from build123d import *

# Parameters (mm, degrees)
SKETCH2_W                       = 42.4
SKETCH2_H                       = 76
SKETCH2_W_2                     = 38.4
SKETCH2_H_2                     = 72
BOSS_EXTRUDE4_DEPTH             = 32
SKETCH1_W                       = 42.4
SKETCH1_H                       = 30
SKETCH1_R                       = 3
BOSS_EXTRUDE1_DEPTH             = 2
SKETCH4_W                       = 56
SKETCH4_H                       = 30
SKETCH4_R                       = 1
BOSS_EXTRUDE5_DEPTH             = 2
SKETCH5_R                       = 1
CUT_EXTRUDE1_DEPTH              = 2
SKETCH9_W                       = 20
SKETCH9_H                       = 1
SKETCH11_W                      = 4.25
SKETCH11_H                      = 3
BOSS_EXTRUDE7_DEPTH             = 25
BOSS_EXTRUDE7_DIRECTION_2_REACH = 97.707
SKETCH12_R                      = 2
CUT_EXTRUDE2_DEPTH              = 25
CHAMFER1_SIZE                   = 1
BOSS_EXTRUDE8_DEPTH             = 2


with BuildPart() as part:
    # Sketch2 → Boss-Extrude4 (new body)
    with BuildSketch(Plane(origin=(0, 0, 0), x_dir=(1, 0, 0), z_dir=(0, 1, 0))):
        with Locations((19.2, 36)):
            Rectangle(SKETCH2_W, SKETCH2_H)
        with Locations((19.2, 36)):
            Rectangle(SKETCH2_W_2, SKETCH2_H_2, mode=Mode.SUBTRACT)
    extrude(amount=BOSS_EXTRUDE4_DEPTH)



with BuildPart() as body_2:
    # Sketch1 → Boss-Extrude1 (new body)
    with BuildSketch(Plane(origin=(0, 32, 0), x_dir=(1, 0, 0), z_dir=(0, 1, 0))):
        with Locations((19.2, 13)):
            Rectangle(SKETCH1_W, SKETCH1_H)
        with Locations(Location((4.2, 3, 0), (0, 0, 270))):
            Circle(SKETCH1_R, mode=Mode.SUBTRACT)
        with Locations(Location((34.2, 3, 0), (0, 0, 90))):
            Circle(SKETCH1_R, mode=Mode.SUBTRACT)
        with Locations(Location((34.2, 23, 0), (0, 0, 270))):
            Circle(SKETCH1_R, mode=Mode.SUBTRACT)
        with Locations(Location((4.2, 23, 0), (0, 0, 90))):
            Circle(SKETCH1_R, mode=Mode.SUBTRACT)
    extrude(amount=BOSS_EXTRUDE1_DEPTH)


with BuildPart() as part_1:
    add(part.part)

    add(body_2.part)  # Boss-Extrude5 merges body 2
    # Sketch4 → Boss-Extrude5 (add)
    with BuildSketch(Plane(origin=(0, 32, 0), x_dir=(1, 0, 0), z_dir=(0, 1, 0))):
        with Locations((19.2, 43)):
            Rectangle(SKETCH4_W, SKETCH4_H)
        with Locations(Location((-3.8, 33, 0), (0, 0, 270))):
            Circle(SKETCH4_R, mode=Mode.SUBTRACT)
        with Locations(Location((-3.8, 53, 0), (0, 0, 90))):
            Circle(SKETCH4_R, mode=Mode.SUBTRACT)
        with Locations(Location((42.2, 53, 0), (0, 0, 270))):
            Circle(SKETCH4_R, mode=Mode.SUBTRACT)
        with Locations(Location((42.2, 33, 0), (0, 0, 90))):
            Circle(SKETCH4_R, mode=Mode.SUBTRACT)
    extrude(amount=BOSS_EXTRUDE5_DEPTH)

    # Sketch5 → Cut-Extrude1 (cut)
    with BuildSketch(Plane.ZY.offset(2)):
        with Locations((-7.7, 5)):
            Circle(SKETCH5_R)
        with Locations((-7.7, 27)):
            Circle(SKETCH5_R)
        with Locations((-64.3, 27)):
            Circle(SKETCH5_R)
        with Locations((-64.3, 5)):
            Circle(SKETCH5_R)
    extrude(amount=-CUT_EXTRUDE1_DEPTH, mode=Mode.SUBTRACT)

    # Sketch9 → Revolve1 (revolve)
    with BuildSketch(Plane(origin=(0, 0, 0), x_dir=(0, 0, -1), z_dir=(1, 0, 0))):
        with Locations((46, 0.5)):
            Rectangle(SKETCH9_W, SKETCH9_H)
        with Locations((26, 0.5)):
            Rectangle(SKETCH9_W, SKETCH9_H)
    revolve1 = revolve(axis=Axis((0, 1, -56), (0, 0, 1)))

    # Mirror1: Revolve1 across plane
    add(revolve1.mirror(Plane(origin=(19.2, 0, 0), x_dir=(0, 0, 1), z_dir=(1, 0, 0))))

    # Sketch11 → Boss-Extrude7 (add)
    with BuildSketch(Plane(origin=(0, 0, -74), x_dir=(-1, 0, 0), z_dir=(0, 0, -1))):
        Polygon((-14.95, 0), (2, 0), (2, 2), (-40.4, 2), (-40.4, 0), (-23.45, 0), (-19.2, 0), align=None)
        with Locations((-21.325, -1.5)):
            Rectangle(SKETCH11_W, SKETCH11_H)
        with Locations((-17.075, -1.5)):
            Rectangle(SKETCH11_W, SKETCH11_H)
    extrude(amount=BOSS_EXTRUDE7_DEPTH)

    # Boss-Extrude7 direction 2: up to this face of the body (flat: up to its plane)
    boss_extrude7_direction_2_end = Plane(part_1.part.faces().sort_by_distance((19.2, 16, -72))[0])
    # Sketch11 → Boss-Extrude7 direction 2 (add, up to the picked face)
    with BuildSketch(Plane(origin=(0, 0, -74), x_dir=(-1, 0, 0), z_dir=(0, 0, -1)), mode=Mode.PRIVATE) as boss_extrude7_direction_2_sk1:
        Polygon((-14.95, 0), (2, 0), (2, 2), (-40.4, 2), (-40.4, 0), (-23.45, 0), (-19.2, 0), align=None)
    boss_extrude7_direction_2_tool1 = split(extrude(boss_extrude7_direction_2_sk1.sketch, amount=-BOSS_EXTRUDE7_DIRECTION_2_REACH, mode=Mode.PRIVATE), bisect_by=boss_extrude7_direction_2_end, keep=Keep.BOTH, mode=Mode.PRIVATE)
    # Sketch11 → Boss-Extrude7 direction 2 (add, up to the picked face)
    with BuildSketch(Plane(origin=(0, 0, -74), x_dir=(-1, 0, 0), z_dir=(0, 0, -1)), mode=Mode.PRIVATE) as boss_extrude7_direction_2_sk2:
        with Locations((-21.325, -1.5)):
            Rectangle(SKETCH11_W, SKETCH11_H)
    boss_extrude7_direction_2_tool2 = split(extrude(boss_extrude7_direction_2_sk2.sketch, amount=-BOSS_EXTRUDE7_DIRECTION_2_REACH, mode=Mode.PRIVATE), bisect_by=boss_extrude7_direction_2_end, keep=Keep.BOTH, mode=Mode.PRIVATE)
    # Sketch11 → Boss-Extrude7 direction 2 (add, up to the picked face)
    with BuildSketch(Plane(origin=(0, 0, -74), x_dir=(-1, 0, 0), z_dir=(0, 0, -1)), mode=Mode.PRIVATE) as boss_extrude7_direction_2_sk3:
        with Locations((-17.075, -1.5)):
            Rectangle(SKETCH11_W, SKETCH11_H)
    boss_extrude7_direction_2_tool3 = split(extrude(boss_extrude7_direction_2_sk3.sketch, amount=-BOSS_EXTRUDE7_DIRECTION_2_REACH, mode=Mode.PRIVATE), bisect_by=boss_extrude7_direction_2_end, keep=Keep.BOTH, mode=Mode.PRIVATE)
    add(boss_extrude7_direction_2_tool1.solids().sort_by(Axis((19.2, 1, -74), (0, 0, 1)))[0])
    add(boss_extrude7_direction_2_tool2.solids().sort_by(Axis((21.325, -1.5, -74), (0, 0, 1)))[0])
    add(boss_extrude7_direction_2_tool3.solids().sort_by(Axis((17.075, -1.5, -74), (0, 0, 1)))[0])

    # Sketch12 → Cut-Extrude2 (cut)
    with BuildSketch(Plane(origin=(0, 2, 0), x_dir=(1, 0, 0), z_dir=(0, 1, 0))):
        with Locations(Location((19.2, 86.5, 0), (0, 0, 270))):
            Circle(SKETCH12_R)
    extrude(amount=-CUT_EXTRUDE2_DEPTH, mode=Mode.SUBTRACT)

    # Chamfer1
    chamfer1_edges = [part_1.edges().sort_by_distance(p)[0] for p in [
        (23.45, -3, -85.5),
        (14.95, -3, -85.5),
    ]]
    chamfer(chamfer1_edges, length=CHAMFER1_SIZE)

    # Sketch13 → Boss-Extrude8 (add)
    with BuildSketch(Plane(origin=(0, 34, 0), x_dir=(1, 0, 0), z_dir=(0, 1, 0))):
        Polygon((40.4, -2), (47.2, 28), (40.4, 28), align=None)
        Polygon((-8.8, 28), (-2, 28), (-2, -2), align=None)
    extrude(amount=-BOSS_EXTRUDE8_DEPTH)


solid = part_1.part
Input: part model. Units: mm. Frame: model coordinates. A direction names the side the tool comes from. Give positions to 0.01 mm unless a question says otherwise; leave off trailing zeros. Write each loop counter-clockwise with the first axis right and the second up, starting at its lowest first coordinate (ties: lowest second). Pieces come first, ordered by that corner, then holes. Notation, with made-up numbers: M -19,-6.5 L 8,-6.5 A25 ccw 8,28.5 Z; hole C -19.75,47.5 d8. An arc over 180 degrees is marked long. Write item = value, one per line. Start each with the question number.
1) Cut plane A-A on z = -33. Return the cut outline in (x, y), then the cut area to 3 significant figures.
2) Cut plane D-D on y = 5. Return the cut outline in (x, z).
3) Cut plane B-B on y = 16.5. Return the cut outline in (x, z).
4) First-contact query: pin 1 Ø19 at (x, z) = (22.5, -40.5) entering from -Y; pin 2 Ø10 at (x, y) = (13, 21) entering from -Z; pin 3 Ø1.2 at (y, z) = (27, -7.7) entering from -X; pin 4 Ø5 at (x, z) = (4.2, -23) entering from +Y. Flat tips, straight axial feed; report the tip coordinate or a pass-through.
5) Reachability of faces 4 (the flat face through (38.4, 16, -35)), 5 (the cylindrical face through (-1.014, 5.3, -6.746)), 6 (the flat face through (-2, 16, -37)), 7 (the flat face through (40.4, 16, -37)) from +Z, -Z, +X, -X, +Y, -Y: full face, straight path, thin tool, end or side. Return the list, or none.
6) Material intervals for line 1 along X through (y, z) = (32.75, -33); line 2 along X through (y, z) = (26.5, -68); line 3 along Z through (x, y) = (21, 31), sorted ascending. Write a range as [from, to].
7) Draft query along Z for faces 1 (the flat face through (19, 33, -58)), 2 (the flat face through (24, 0, -74)), 3 (the flat face through (0, 16, -35)). Return one class per face: +Z half, -Z half, draft (parallel to the pull), parting line (faces both ways), or undercut.
8) Cut plane C-C on x = 10.5. Return the cut outline in (y, z).
Solved:
q1.outline = M -8.8,32 L -4.8,32 L -4.8,34 L -8.8,34 Z; M -2.8,32 L -2,32 L -2,0 L 0,0 A1 ccw 0,2 L 0,32 L 38.4,32 L 38.4,2 A1 ccw 38.4,0 L 40.4,0 L 40.4,32 L 41.2,32 L 41.2,34 L -2.8,34 Z; M 43.2,32 L 47.2,32 L 47.2,34 L 43.2,34 Z
q1.area = 235 mm2
q2.outline = M -2,-74 L 40.4,-74 L 40.4,2 L -2,2 L -2,-6.7 L 0,-6.7 L 0,0 L 38.4,0 L 38.4,-72 L 0,-72 L 0,-65.3 L -2,-65.3 Z; M -2,-63.3 L 0,-63.3 L 0,-8.7 L -2,-8.7 Z
q3.outline = M -2,-74 L 40.4,-74 L 40.4,2 L -2,2 Z; hole M 0,-72 L 38.4,-72 L 38.4,0 L 0,0 Z
q4.pin_1 = 32
q4.pin_2 = -74
q4.pin_3 = 38.4
q4.pin_4 = through
q5.face_4 = none
q5.face_5 = -X
q5.face_6 = +Z, -Z, -X, -Y
q5.face_7 = +Z, -Z, +X, -Y
q6.line_1 = [-8.8, -4.8], [-2.8, 41.2], [43.2, 47.2]
q6.line_2 = [-2, 0], [38.4, 40.4]
q6.line_3 = [-74, -72], [0, 2]
q7.face_1 = -Z half
q7.face_2 = draft
q7.face_3 = undercut
q8.outline = M 0,-99 L 2,-99 L 2,-74 L 32,-74 L 32,-72 L 0,-72 Z; M 0,0 L 32,0 L 32,-58 L 34,-58 L 34,2 L 0,2 Z
